For this review, take the finished solid that the model builds, in its own axes (mm). A direction names the side the tool comes from. Round coordinates to 2 decimals unless told otherwise and drop trailing zeros. Order: outer loops, then holes, each group sorted by start corner. A loop starts at its lowest first (then second) coordinate and runs counter-clockwise, first axis right, second up. Notation, with made-up numbers: M 19,-11 L 69,-11 A9 cw 69,-2 Z; hole C 17,34.25 d11. An arc over 180 degrees is marked long. Use a Markdown table: item, result.
Autodesk Inventor part; units mm, degrees
ref_plane "YZ Plane" through (0, 0, 0) normal (1, 0, 0) x (0, 1, 0)
ref_plane "XZ Plane" through (0, 0, 0) normal (0, 1, 0) x (-1, 0, 0)
ref_plane "XY Plane" through (0, 0, 0) normal (0, 0, 1) x (1, 0, 0)
sketch "スケッチ1" plane through (0, 0, 0) normal (0, 0, 1) x (1, 0, 0)
  circle A0 centre (0, 0) radius 1.65
  dimension "d0" = 3.3
extrude "押し出し1" add sketch "スケッチ1" along normal blind 16
sketch "スケッチ2" plane through (0, 0, 16) normal (0, 0, 1) x (1, 0, 0)
  circle A0 centre (0, 0) radius 4
  dimension "d3" = 8
extrude "押し出し2" add sketch "スケッチ2" against normal blind 2.3
chamfer "面取り1" distance 2.3 angle 45 1 edges at (-4, 0, 13.7)
thread "ねじ1"
properties part number "ネジ皿m4,16" material "鋼、高強度、低合金"
Q1. Add section C-C (z = 1.5). Write out the cut boundary in (x, y).
Determined:
| item | result |
|---|---|
| outline | C 0,0 d3.3 |
Q2. Add section D-D (z = 15.25). Write out the cut boundary in (x, y).
Determined:
| item | result |
|---|---|
| outline | C 0,0 d6.5 |
Q3. Wall thickness on line 1 along X through (y, z) = (0, 10.5); line 2 along Z through (x, y) = (1.5, -1.75); line 3 along Y through (x, z) = (-1.75, 15): over which ranges is each line inside the solid? List them lowest first. Write a range as [from, to].
Determined:
| item | result |
|---|---|
| line 1 | x = [-1.65, 1.65] |
| line 2 | z = [14.3, 16] |
| line 3 | y = [-2.44, 2.44] |
Q4. Clearance check with flat-ended pins moving along their axes: pin 1 (1.5 mm diameter, centred on x = -3, z = 4.5, fed in from -Y); pin 2 (1.5 mm diameter, centred on x = -2.5, y = -1, fed in from -Z); pin 3 (4 mm diameter, centred on y = -3, z = 10.5, fed in from +X). State where each tip first meets the part, or that it passes through.
Determined:
| item | result |
|---|---|
| pin 1 | passes through |
| pin 2 | stops at z = 13.94 |
| pin 3 | stops at x = 1.31 |
Q5. Machinability: for faces 1 (the cylindrical face through (-1.216, -1.115, 6.754)), 2 (the flat face through (0, 0, 16)), which of the approach directions +Z, -Z, +X, -X, +Y, -Y give a long, thin tool a straight path to every point of the face, cutting with its end or side? Answer none if there is none.
Determined:
| item | result |
|---|---|
| face 1 | -Z |
| face 2 | +Z, +X, -X, +Y, -Y |
